from build123d import *

# Parameters (mm, degrees)
AUFSATZ_LINEAR_AUSTRAGEN1_DEPTH = 2.5
VERRUNDUNG1_R                   = 10
VERRUNDUNG2_R                   = 10
VERRUNDUNG3_R                   = 2
VERRUNDUNG4_R                   = 0.5
VERRUNDUNG5_R                   = 10


with BuildPart() as part:
    # Skizze1 → Aufsatz-Linear austragen1 (new, symmetric)
    with BuildSketch(Plane.XY):
        Polygon((46.512935857, 2.5), (55.211178367, 14.470305023), (72.222811922, 10.746349053), (59.213582381, 7.260536503), (62.060591877, -3.364647586), (74.617627619, 0), (62.199292585, -11.609692287), (48.474059835, -5.5), (-46.512935857, -5.5), (-52.459487047, -12.797272415), (-67.79418193, -9.659258263), (-56.203072015, -6.553429722), (-58.791262466, 3.105828541), (-70.382372381, 0), (-58.671144129, 10.384947415), (-46.512935857, 2.5), align=None)
    extrude(amount=AUFSATZ_LINEAR_AUSTRAGEN1_DEPTH, both=True)

    # Verrundung1
    verrundung1_edges = [part.edges().sort_by_distance(p)[0] for p in [
        (-52.459487047, -12.797272415, 0),
        (-58.671144129, 10.384947415, 0),
    ]]
    fillet(verrundung1_edges, radius=VERRUNDUNG1_R)

    # Verrundung2
    verrundung2_edges = [part.edges().sort_by_distance(p)[0] for p in [
        (62.199292585, -11.609692287, 0),
        (55.211178367, 14.470305023, 0),
    ]]
    fillet(verrundung2_edges, radius=VERRUNDUNG2_R)

    # Verrundung3
    verrundung3_edges = [part.edges().sort_by_distance(p)[0] for p in [
        (59.213582381, 7.260536503, 0),
        (62.060591877, -3.364647586, 0),
        (-56.203072015, -6.553429722, 0),
        (-58.791262466, 3.105828541, 0),
    ]]
    fillet(verrundung3_edges, radius=VERRUNDUNG3_R)

    # Verrundung4
    verrundung4_edges = [part.edges().sort_by_distance(p)[0] for p in [
        (72.222811922, 10.746349053, 0),
        (74.617627619, 0, 0),
        (-67.79418193, -9.659258263, 0),
        (-70.382372381, 0, 0),
    ]]
    fillet(verrundung4_edges, radius=VERRUNDUNG4_R)

    # Verrundung5
    verrundung5_edges = [part.edges().sort_by_distance(p)[0] for p in [
        (46.512935857, 2.5, 0),
        (48.474059835, -5.5, 0),
        (-46.512935857, -5.5, 0),
        (-46.512935857, 2.5, 0),
    ]]
    fillet(verrundung5_edges, radius=VERRUNDUNG5_R)


solid = part.part
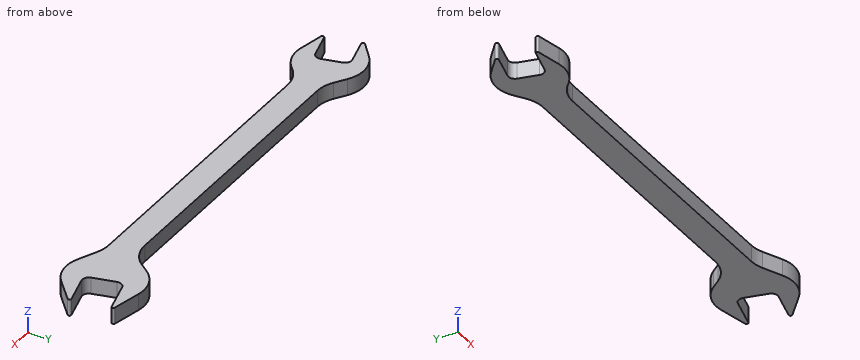
Input: part model. Units: mm. Frame: model coordinates. Coordinates: 2 decimals unless noted, no trailing zeros. Loops run counter-clockwise (first coordinate to the right, second up) from the corner with the lowest first, then second, coordinate; pieces in that order, holes last. Notation, with made-up numbers: (85.5, -11.5) -> (108.5, -11.5) arc R16 cw to (108.5, 19.5) -> close; hole circle Ø8 at (-2, 44.25). An arc over 180 degrees is marked (long way). One line per item, written item: value.
(1) Ray query, line 1 along Y through (x, z) = (-39, 1.9); line 2 along X through (y, z) = (7, 0.4); line 3 along X through (y, z) = (0.5, 2.05). Return the intervals inside material, ascending.
Answer below:
line 1: y = -5.5 to 2.5
line 2: x = -61.77 to -53.68, 49.78 to 60.03
line 3: x = -58.09 to 61.03
(2) Pin query (flat end, axial travel): pin 1 Ø2 at (y, z) = (-6, -1.5) entering from +X; pin 2 Ø2.5 at (x, z) = (12.5, -1) entering from +Y; pin 3 Ø1.5 at (x, z) = (13.5, -0.5) entering from -Y. Return the tip coordinate at first contact, or that it passes through.
Answer below:
pin 1: stops at x = 69.27
pin 2: stops at y = 2.5
pin 3: stops at y = -5.5
(3) Cut plane A-A (x = -1.5). Output: boundary loops of the cut face in (y, z).
Answer below:
outline: (-5.5, -2.5) -> (2.5, -2.5) -> (2.5, 2.5) -> (-5.5, 2.5) -> close
